CAD build for the part. Positions are in the model's coordinates, mm. Face numbers are marked on the shaded views. A direction names the side the tool comes from. Give positions to 0.01 mm unless a question says otherwise; leave off trailing zeros. Loops run counter-clockwise (first coordinate to the right, second up) from the corner with the lowest first, then second, coordinate; pieces in that order, holes last. Notation, with made-up numbers: M -18.75,69 L 15.25,69 A19 cw 15.25,73 Z; hole C 80.25,50.5 d2. An arc over 180 degrees is marked long. Answer as CSV lines item,"result".
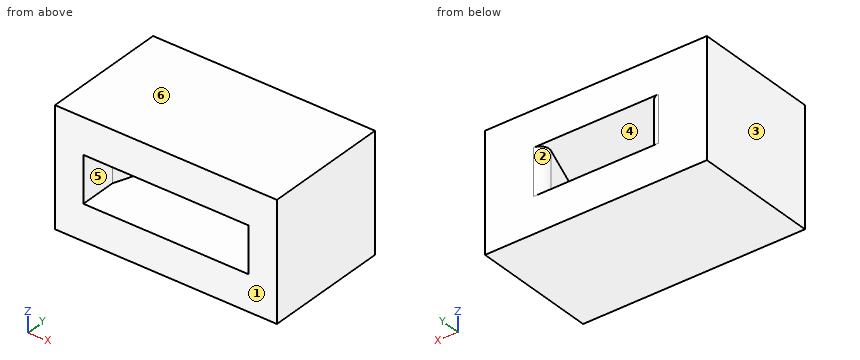
Autodesk Fusion 360 part; units mm, degrees
sketch "Sketch1" plane through (0, 0, 0) normal (0, 0, 1) x (1, 0, 0)
  line L0 (0, 0) -> (25, 0)
  line L1 (25, 0) -> (25, -15.2)
  line L2 (25, -15.2) -> (0, -15.2)
  line L3 (0, -15.2) -> (0, 0)
  line L4 (7.25, 0) -> (3.2, -11)
  line L5 (17.75, 0) -> (21.8, -11)
  line L6 (3.2, -11) -> (3.2, -15.2)
  line L7 (21.8, -11) -> (21.8, -15.2)
  line L8 (3.2, -15.2) -> (21.8, -15.2) construction
  line L9 (12.5, -8.3) -> (25, -8.3) construction
  line L10 (12.5, -8.3) -> (0, -8.3) construction
  line L11 (0, 0) -> (7.25, 0) construction
  line L12 (17.75, 0) -> (25, 0) construction
  line L13 (36.4201, 0) -> (32.3701, -11.4) construction
  line L14 (32.3701, -11.4) -> (32.3701, -15.2) construction
  line L15 (32.3701, -15.2) -> (50.1701, -15.2) construction
  line L16 (50.1701, -15.2) -> (50.1701, -11.4) construction
  line L17 (50.1701, -11.4) -> (46.1201, 0) construction
  line L18 (36.4201, 0) -> (46.1201, 0) construction
  dimension "d1" = 25
  dimension "d2" = 15.2
  dimension "d3" = 10.5
  dimension "d5" = 18.6
  dimension "d10" = 11
  dimension "d14" = 8.3
  dimension "d26" = 3.8
  dimension "d27" = 17.8
  dimension "d28" = 9.7
  dimension "d29" = 15.2
extrude "Extrude1" add sketch "Sketch1" against normal blind 4 makes body 1
extrude "Extrude2" add sketch "Sketch1" along normal blind 5.2 contours L0 L2 L3 L4 L6 | L0 L1 L2 L5 L7 bodies 1
extrude "Extrude3" add sketch "Sketch1" along normal blind 4 from surface at 5.2 separate body makes body 2
combine "Combine1" operation add target body 1 tool bodies 2
extrude "Extrude5" cut 1 faces at (22.5833, 0, 1.7333) along direction (0, -1, 0) blind 1 on bodies 1 bodies 1
fillet "Fillet2" radius 1 2 edges at (6.8818, -1, 2.6) (18.1182, -1, 2.6) on bodies 1
equation "d3 = 9.7 mm + 0.8 mm"
equation "d5 = 17.8 mm + 0.8 mm"
equation "d14 = 8.4 mm - 0.1 mm"
equation "d17 = 5 mm + 0.2 mm"
1) Band-saw the part on A-A on z = 4.25. Give the cut face in (x, y), and give its area (3 significant figures).
Answer below:
outline,"M 0,-15.2 L 3.2,-15.2 L 3.2,-11 L 6.39,-2.35 A1 ccw 5.45,-1 L 0,-1 Z; M 18.61,-2.35 L 21.8,-11 L 21.8,-15.2 L 25,-15.2 L 25,-1 L 19.55,-1 A1 ccw Z"
area,"127 mm^2"
2) Which spindle directions (+Z, -Z, +X, -X, +Y, -Y) get a long thin tool onto all of the face, cutting with end or side? Do the marked faces 1 and 2. Say none if no direction does.
Answer below:
face 1,"+Z, -Z, +X, -X, -Y"
face 2,"none"
3) Band-saw the part on B-B on x = 16.25. Give the cut face in (y, z), and give its area (3 significant figures).
Answer below:
outline,"M -15.2,-4 L -1,-4 L -1,0 L -15.2,0 Z; M -15.2,5.2 L -1,5.2 L -1,9.2 L -15.2,9.2 Z"
area,"114 mm^2"
4) Mould opens along X. For the marked faces 3, 4, 5 and 6 say: +X half, -X half, draft (parallel to the pull), parting line (faces both ways), or undercut.
Answer below:
face 3,"-X half"
face 4,"undercut"
face 5,"undercut"
face 6,"draft"
5) Drill centre lines: line 1 (Z direction, x = 16.75, y = -9.25); line 2 (X direction, y = -11.5, z = 4.5); line 3 (X direction, y = -3, z = 2.75). Where is each one in solid material? Low to high. Write a range as from..to.
Answer below:
line 1,"z = -4..0, 5.2..9.2"
line 2,"x = 0..3.2, 21.8..25"
line 3,"x = 0..6.15, 18.85..25"
6) Band-saw the part on C-C on y = -12.5. Give the cut face in (x, z), and give its area (3 significant figures).
Answer below:
outline,"M 0,-4 L 25,-4 L 25,9.2 L 0,9.2 Z; hole M 3.2,0 L 21.8,0 L 21.8,5.2 L 3.2,5.2 Z"
area,"233 mm^2"
7) Band-saw the part on D-D on y = -3.25. Give the cut face in (x, z), and give its area (3 significant figures).
Answer below:
outline,"M 0,-4 L 25,-4 L 25,9.2 L 0,9.2 Z; hole M 6.05,0 L 18.95,0 L 18.95,5.2 L 6.05,5.2 Z"
area,"263 mm^2"
